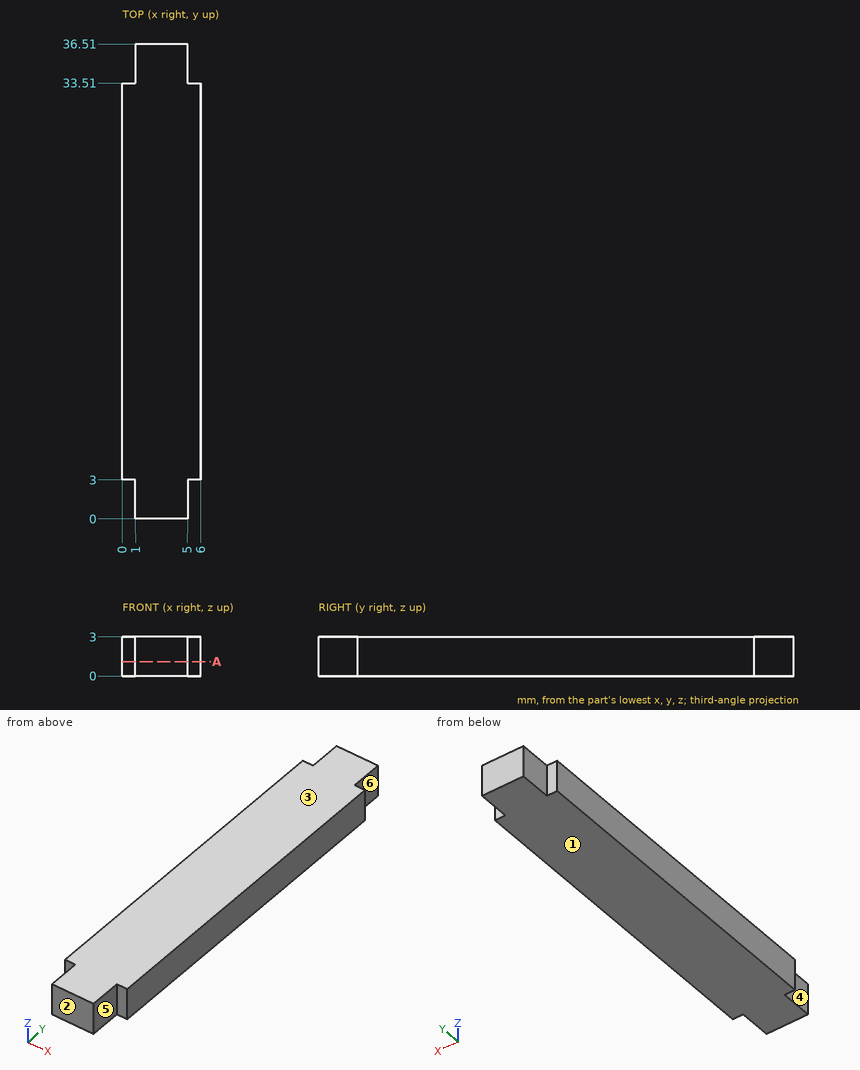
Design review of the part shown in the three views and the two pictorial views. Dimensions are in mm from the part's minimum x, y and z. A direction names the side the tool comes from. Round coordinates to 2 decimals unless told otherwise and drop trailing zeros. Loops run counter-clockwise (first coordinate to the right, second up) from the corner with the lowest first, then second, coordinate; pieces in that order, holes last.
Q1. Add section A-A on z = 1.1. Write out the cut boundary in (x, y).
Result sheet:
outline: (0, 3) - (1, 3) - (1, 0) - (5, 0) - (5, 3) - (6, 3) - (6, 33.51) - (5, 33.51) - (5, 36.51) - (1, 36.51) - (1, 33.51) - (0, 33.51) - close
Q2. Machinability: for the marked faces 4, 5 and 6, which of the approach directions +Z, -Z, +X, -X, +Y, -Y give a long, thin tool a straight path to every point of the face, cutting with its end or side? Answer none if there is none.
Result sheet:
face 4: +Z, -Z, -X, -Y
face 5: +Z, -Z, +X, -Y
face 6: +Z, -Z, +X, +Y
Q3. Insertion check: pin 1 Ø1.1 at (x, z) = (5.5, 1.5) entering from -Y; pin 2 Ø0.8 at (x, z) = (0.5, 1.5) entering from -Y; pin 3 Ø1.5 at (y, z) = (1, 2) entering from +X; pin 4 Ø1.5 at (y, z) = (35, 1.5) entering from -X. Each pin has a flat end and moves straight along its axis. Give the tip position at first contact, or say it passes through.
Result sheet:
pin 1: stops at y = 0
pin 2: stops at y = 3
pin 3: stops at x = 5
pin 4: stops at x = 1
Q4. Mouldability with a two-part tool opening along Z and no side actions: class the marked faces 1, 2 and 3 as +Z half, -Z half, draft (parallel to the pull), parting line (faces both ways), or undercut.
Result sheet:
face 1: -Z half
face 2: draft
face 3: +Z half
Q5. To check wall thickness, follow line 1 along Y through (x, z) = (5.6, 2.75); line 2 along X through (y, z) = (2, 2.45). State the ranges of each line that lie inside material, in increasing order.
Result sheet:
line 1: y = 3 to 33.51
line 2: x = 1 to 5
